Here's how the part is built. I have some questions about the finished solid (model axes, mm). A direction names the side the tool comes from. Round coordinates to 2 decimals unless told otherwise and drop trailing zeros. Order: outer loops, then holes, each group sorted by start corner. A loop starts at its lowest first (then second) coordinate and runs counter-clockwise, first axis right, second up. Notation, with made-up numbers: (7.25, 71.5) - (66.25, 71.5) arc R14 ccw to (66.25, 82.5) - close; hole circle Ø3 at (59.5, -36.75). An arc over 180 degrees is marked (long way). Answer as a JSON object with one key per item and string values.
```python
from build123d import *

# Parameters (mm, degrees)
SKETCH1_R           = 1.1
BOSS_EXTRUDE1_DEPTH = 5
SKETCH2_W           = 16
SKETCH2_H           = 12
BOSS_EXTRUDE2_DEPTH = 15
CUT_EXTRUDE1_START  = -5.5
SKETCH3_W           = 9
SKETCH3_H           = 15.5
CUT_EXTRUDE1_DEPTH  = 9.5
SKETCH4_R           = 1
CUT_EXTRUDE2_DEPTH  = 16
FILLET2_R           = 0.5
SKETCH5_R           = 1.9
CUT_EXTRUDE3_DEPTH  = 1
FILLET3_R           = 1
CUT_EXTRUDE4_START  = -0.5
SKETCH6_R           = 2
CUT_EXTRUDE4_DEPTH  = 5.5
FILLET4_R           = 3
FILLET5_R           = 0.5


with BuildPart() as part:
    # Sketch1 → Boss-Extrude1 (new body)
    with BuildSketch(Plane.XY):
        with BuildLine():
            ThreePointArc((0, 4.5), (-4.5, 0), (0, -4.5))
            Line((0, -4.5), (50, -4.5))
            Line((50, -4.5), (50, 4.5))
            Line((50, 4.5), (0, 4.5))
        make_face()
        Circle(SKETCH1_R, mode=Mode.SUBTRACT)
    extrude(amount=BOSS_EXTRUDE1_DEPTH)

    # Sketch2 → Boss-Extrude2 (add)
    with BuildSketch(Plane(origin=(0, 4.5, 0), x_dir=(1, 0, 0), z_dir=(0, 1, 0))):
        with Locations((58, -6)):
            Rectangle(SKETCH2_W, SKETCH2_H)
    extrude(amount=-BOSS_EXTRUDE2_DEPTH)

    # Sketch3 → Cut-Extrude1 (cut)
    with BuildSketch(Plane(origin=(0, 4.5, 0), x_dir=(1, 0, 0), z_dir=(0, 1, 0)).offset(CUT_EXTRUDE1_START)):
        with Locations((57.5, -4.25)):
            Rectangle(SKETCH3_W, SKETCH3_H)
    extrude(amount=-CUT_EXTRUDE1_DEPTH, mode=Mode.SUBTRACT)

    # Sketch4 → Cut-Extrude2 (cut)
    with BuildSketch(Plane(origin=(66, 0, 0), x_dir=(0, 0, -1), z_dir=(1, 0, 0))):
        with Locations((-6, -6.5)):
            Circle(SKETCH4_R)
    extrude(amount=-CUT_EXTRUDE2_DEPTH, mode=Mode.SUBTRACT)

    # Fillet2
    fillet2_edges = [part.edges().sort_by_distance(p)[0] for p in [
        (53, -6.5, 7),
    ]]
    fillet(fillet2_edges, radius=FILLET2_R)

    # Sketch5 → Cut-Extrude3 (cut)
    with BuildSketch(Plane(origin=(66, 0, 0), x_dir=(0, 0, -1), z_dir=(1, 0, 0))):
        with Locations((-6, -6.5)):
            Circle(SKETCH5_R)
    extrude(amount=-CUT_EXTRUDE3_DEPTH, mode=Mode.SUBTRACT)

    # Fillet3
    fillet3_edges = [part.edges().sort_by_distance(p)[0] for p in [
        (53, -10.5, 6),
        (62, -10.5, 6),
        (62, -5.75, 0),
        (53, -5.75, 0),
        (53, -5.75, 12),
        (62, -5.75, 12),
    ]]
    fillet(fillet3_edges, radius=FILLET3_R)

    # Sketch6 → Cut-Extrude4 (cut)
    with BuildSketch(Plane.ZY.offset(-50).offset(CUT_EXTRUDE4_START)):
        with Locations((6, -6.5)):
            Circle(SKETCH6_R)
    extrude(amount=CUT_EXTRUDE4_DEPTH, mode=Mode.SUBTRACT)

    # Fillet4
    # the kernel refuses this fillet: 3 mm, written as the material it takes off along each edge
    with BuildSketch(Plane(origin=(53, -7.5, 3), x_dir=(0, -1, 0), z_dir=(0, 0, 1))) as fillet4_piece_1:
        with BuildLine():
            CenterArc((2, -1), 1, 0, 90)
            Line((3, -1), (3, 0))
            Line((3, 0), (2, 0))
        make_face()
    revolve(axis=Axis((53, -7.5, 3), (1, 0, 0)), revolution_arc=90, mode=Mode.SUBTRACT)
    with BuildSketch(Plane(origin=(53, -7.5, 9), x_dir=(0, 0, 1), z_dir=(0, 1, 0))) as fillet4_piece_2:
        with BuildLine():
            CenterArc((2, -1), 1, 0, 90)
            Line((3, -1), (3, 0))
            Line((3, 0), (2, 0))
        make_face()
    revolve(axis=Axis((53, -7.5, 9), (1, 0, 0)), revolution_arc=90, mode=Mode.SUBTRACT)
    with BuildSketch(Plane(origin=(62, -7.5, 9), x_dir=(0, -1, 0), z_dir=(0, 0, -1))) as fillet4_piece_3:
        with BuildLine():
            CenterArc((2, -1), 1, 0, 90)
            Line((3, -1), (3, 0))
            Line((3, 0), (2, 0))
        make_face()
    revolve(axis=Axis((62, -7.5, 9), (-1, 0, 0)), revolution_arc=90, mode=Mode.SUBTRACT)
    with BuildSketch(Plane(origin=(62, -7.5, 3), x_dir=(0, 0, -1), z_dir=(0, 1, 0))) as fillet4_piece_4:
        with BuildLine():
            CenterArc((2, -1), 1, 0, 90)
            Line((3, -1), (3, 0))
            Line((3, 0), (2, 0))
        make_face()
    revolve(axis=Axis((62, -7.5, 3), (-1, 0, 0)), revolution_arc=90, mode=Mode.SUBTRACT)
    with BuildSketch(Plane(origin=(62, -10.5, 0), x_dir=(0, 1, 0), z_dir=(1, 0, 0)), Plane(origin=(73.5, -10.5, 12), x_dir=(0, 1, 0), z_dir=(-1, 0, 0))) as fillet4_piece_5:
        with BuildLine():
            CenterArc((FILLET4_R, FILLET4_R), FILLET4_R, 180, 90)
            Line((0, FILLET4_R), (0, 0))
            Line((0, 0), (FILLET4_R, 0))
        make_face()
    extrude(amount=11.5, mode=Mode.SUBTRACT)
    with BuildSketch(Plane(origin=(53, -10.5, 12), x_dir=(0, 1, 0), z_dir=(-1, 0, 0)), Plane(origin=(42.5, -10.5, 0), x_dir=(0, 1, 0), z_dir=(1, 0, 0))) as fillet4_piece_6:
        with BuildLine():
            CenterArc((FILLET4_R, FILLET4_R), FILLET4_R, 180, 90)
            Line((0, FILLET4_R), (0, 0))
            Line((0, 0), (FILLET4_R, 0))
        make_face()
    extrude(amount=10.5, mode=Mode.SUBTRACT)

    # Fillet5
    fillet5_edges = [part.edges().sort_by_distance(p)[0] for p in [
        (-1.1, 0, 5),
        (-1.1, 0, 0),
    ]]
    fillet(fillet5_edges, radius=FILLET5_R)


solid = part.part
```
1. Thinking about a two-plate mould opening in X: for faces 4 (the face through (53, -4, 6)), 5 (the face through (30, 0, 0)), 6 (the face through (62, -5, 6)), 7 (the face through (65, -7.32, 5.18)), which applies, pulls with the +X half, pulls with the -X half, needs draft (parallel to the pull), parting line crosses it, or undercut?
Responses:
{"face 4": "undercut", "face 5": "needs draft", "face 6": "undercut", "face 7": "pulls with the +X half"}
2. If I drill on L1, parallel to X at y = -1.5, z = 7; L2, parallel to Z at x = 50.25, y = -6.5; L3, parallel to Y at x = 50.2, z = 6, over which ranges is the centre line in solid material (lowest first)? Write a range as [from, to].
Responses:
{"L1": "[50, 53], [62, 66]", "L2": "[0, 4], [8, 12]", "L3": "[-10.5, -8.5], [-4.5, 4.5]"}
3. Imagine slicing it at C-C (y = -6.5). Give the number of separate pieces and of enclosed holes in the cut face, plus the area to 3 significant figures.
Responses:
{"separate pieces": "4", "enclosed holes": "0", "area": "66.2 mm2"}
4. Imagine slicing it at B-B (z = 6). List the corners of the cut face in (x, y) for me, plus the area to 3 significant figures.
Responses:
{"outline": "(50, -10.5) - (52, -10.5) arc R1 ccw to (53, -9.5) - (53, -8) arc R0.5 ccw to (52.5, -7.5) - (50.5, -7.5) - (50.5, -8.5) - (50, -8.5) - close; (50, -4.5) - (50.5, -4.5) - (50.5, -5.5) - (52.5, -5.5) arc R0.5 ccw to (53, -5) - (53, -1) - (62, -1) - (62, -5.5) - (65, -5.5) - (65, -4.6) - (66, -4.6) - (66, 4.5) - (50, 4.5) - close; (62, -9.5) arc R1 ccw to (63, -10.5) - (66, -10.5) - (66, -8.4) - (65, -8.4) - (65, -7.5) - (62, -7.5) - close", "area": "137 mm2"}
5. Imagine slicing it at D-D (x = 3). List the corners of the cut face in (y, z) for me.
Responses:
{"outline": "(-4.5, 0) - (4.5, 0) - (4.5, 5) - (-4.5, 5) - close"}
6. For P1, Ø5.5, axis at x = 16.5, z = 1.5, coming from the -Y side; P2, Ø1, axis at x = 38, y = -2, coming from the +Z side; P3, Ø1.2, axis at y = -6.5, z = 5.5, coming from the -X side; P4, Ø1.8, axis at y = -6.5, z = 6, coming from the -X side, each with a flat end and sliding along its axis, tell me the tip position at first contact or that it passes through.
Responses:
{"P1": "y = -4.5", "P2": "z = 5", "P3": "x = 50.5", "P4": "through"}
7. For faces 1 (the face through (50.3, -7.7, 4.4)), 2 (the face through (65.507, -5.216, 7.4)), 3 (the face through (50, -3, 7)), which set-ups out of +Z, -Z, +X, -X, +Y, -Y let a thin tool reach every point of the face, with its end or its side?
Responses:
{"face 1": "-X", "face 2": "+X", "face 3": "+Z, -X, -Y"}
8. Imagine slicing it at A-A (y = 0). List the corners of the cut face in (x, z) for me.
Responses:
{"outline": "(-4.5, 0) - (-1.6, 0) arc R0.5 ccw to (-1.1, 0.5) - (-1.1, 4.5) arc R0.5 ccw to (-1.6, 5) - (-4.5, 5) - close; (1.1, 0.5) arc R0.5 ccw to (1.6, 0) - (66, 0) - (66, 12) - (50, 12) - (50, 5) - (1.6, 5) arc R0.5 ccw to (1.1, 4.5) - close"}
